Geometry: final body of the model. Coordinates: model frame, mm. A direction names the side the tool comes from. Round coordinates to 2 decimals unless told otherwise and drop trailing zeros. Loops run counter-clockwise (first coordinate to the right, second up) from the corner with the lowest first, then second, coordinate; pieces in that order, holes last. Notation, with made-up numbers: M 42,8.5 L 54,8.5 A30 ccw 54,43.5 Z; hole C 12.25,9 d9. An arc over 180 degrees is marked long. Answer as a JSON object with one key per item and string values.
from build123d import *

# Parameters (mm, degrees)
SKETCH1_W           = 100
SKETCH1_H           = 205
BOSS_EXTRUDE1_DEPTH = 3
SKETCH2_W           = 100
SKETCH2_H           = 20
BOSS_EXTRUDE2_DEPTH = 3
CUT_EXTRUDE1_REACH  = 125.257
SKETCH3_R           = 2
LPATTERN1_COUNT     = 2
LPATTERN1_PITCH     = 80
SKETCH4_W           = 100
SKETCH4_H           = 3
BOSS_EXTRUDE3_DEPTH = 15
CUT_EXTRUDE2_REACH  = 220.559
SKETCH5_R           = 1.5
LPATTERN2_COUNT     = 2
LPATTERN2_PITCH     = 80
SKETCH7_W           = 3
SKETCH7_H           = 15
CUT_EXTRUDE3_DEPTH  = 3
CUT_EXTRUDE4_REACH  = 126.021
SKETCH6_R           = 1.5


with BuildPart() as part:
    # Sketch1 → Boss-Extrude1 (new body)
    with BuildSketch(Plane(origin=(0, 0, 0), x_dir=(1, 0, 0), z_dir=(0, 1, 0))):
        Rectangle(SKETCH1_W, SKETCH1_H)
    extrude(amount=BOSS_EXTRUDE1_DEPTH)

    # Sketch2 → Boss-Extrude2 (add)
    with BuildSketch(Plane(origin=(0, 3, 0), x_dir=(1, 0, 0), z_dir=(0, 1, 0))):
        with Locations((0, 102.5)):
            Rectangle(SKETCH2_W, SKETCH2_H)
    extrude(amount=BOSS_EXTRUDE2_DEPTH)

    # Sketch3 → Cut-Extrude1 (cut, up to next)
    with BuildSketch(Plane(origin=(0, 6, 0), x_dir=(1, 0, 0), z_dir=(0, 1, 0)), mode=Mode.PRIVATE) as cut_extrude1_sk1:
        with Locations(Location((-40, 107.5, 0), (0, 0, 270))):
            Circle(SKETCH3_R)
    cut_extrude1_tool1 = extrude(cut_extrude1_sk1.sketch, amount=-CUT_EXTRUDE1_REACH, mode=Mode.PRIVATE) & part.part
    cut_extrude1 = cut_extrude1_tool1.solids().sort_by_distance((-40, 6, -107.5))[0]
    add(cut_extrude1, mode=Mode.SUBTRACT)

    # LPattern1: Cut-Extrude1 ×2
    with Locations(*[(i * LPATTERN1_PITCH, 0, 0) for i in range(1, LPATTERN1_COUNT)]):
        add(cut_extrude1, mode=Mode.SUBTRACT)

    # Sketch4 → Boss-Extrude3 (add)
    with BuildSketch(Plane(origin=(0, 3, 0), x_dir=(1, 0, 0), z_dir=(0, 1, 0))):
        with Locations((0, -98)):
            Rectangle(SKETCH4_W, SKETCH4_H)
    extrude(amount=BOSS_EXTRUDE3_DEPTH)

    # Sketch5 → Cut-Extrude2 (cut, up to next)
    with BuildSketch(Plane.XY.offset(99.5), mode=Mode.PRIVATE) as cut_extrude2_sk1:
        with Locations((-40, 10.5)):
            Circle(SKETCH5_R)
    cut_extrude2_tool1 = extrude(cut_extrude2_sk1.sketch, amount=-CUT_EXTRUDE2_REACH, mode=Mode.PRIVATE) & part.part
    cut_extrude2 = cut_extrude2_tool1.solids().sort_by_distance((-40, 10.5, 99.5))[0]
    add(cut_extrude2, mode=Mode.SUBTRACT)

    # LPattern2: Cut-Extrude2 ×2
    with Locations(*[(i * LPATTERN2_PITCH, 0, 0) for i in range(1, LPATTERN2_COUNT)]):
        add(cut_extrude2, mode=Mode.SUBTRACT)

    # Sketch7 → Cut-Extrude3 (cut)
    with BuildSketch(Plane(origin=(50, 0, 0), x_dir=(0, 0, -1), z_dir=(1, 0, 0))):
        with Locations((-98, 10.5)):
            Rectangle(SKETCH7_W, SKETCH7_H)
    extrude(amount=-CUT_EXTRUDE3_DEPTH, mode=Mode.SUBTRACT)

    # Sketch6 → Cut-Extrude4 (cut, up to next)
    with BuildSketch(Plane(origin=(0, 3, 0), x_dir=(1, 0, 0), z_dir=(0, 1, 0)), mode=Mode.PRIVATE) as cut_extrude4_sk1:
        with Locations(Location((-46, 13.97, 0), (0, 0, 270))):
            Circle(SKETCH6_R)
    cut_extrude4_tool1 = extrude(cut_extrude4_sk1.sketch, amount=-CUT_EXTRUDE4_REACH, mode=Mode.PRIVATE) & part.part
    # Sketch6 → Cut-Extrude4 (cut, up to next)
    with BuildSketch(Plane(origin=(0, 3, 0), x_dir=(1, 0, 0), z_dir=(0, 1, 0)), mode=Mode.PRIVATE) as cut_extrude4_sk2:
        with Locations(Location((46, 13.97, 0), (0, 0, 270))):
            Circle(SKETCH6_R)
    cut_extrude4_tool2 = extrude(cut_extrude4_sk2.sketch, amount=-CUT_EXTRUDE4_REACH, mode=Mode.PRIVATE) & part.part
    add(cut_extrude4_tool1.solids().sort_by_distance((-46, 3, -13.97))[0], mode=Mode.SUBTRACT)
    add(cut_extrude4_tool2.solids().sort_by_distance((46, 3, -13.97))[0], mode=Mode.SUBTRACT)


solid = part.part
1) Ray query, line 1 (X direction, y = 0.7, z = -13.97); line 2 (X direction, y = 5.1, z = -107.5); line 3 (Y direction, x = 40, z = 97). Return the intervals inside material, ascending.
Results:
{"line 1": "-50 to -47.5, -44.5 to 44.5, 47.5 to 50", "line 2": "-50 to -42, -38 to 38, 42 to 50", "line 3": "0 to 9, 12 to 18"}
2) Section query B-B (x = -27). Return the cut outline in (y, z), and give its area (3 significant figures).
Results:
{"outline": "M 0,-102.5 L 3,-102.5 L 3,-112.5 L 6,-112.5 L 6,-92.5 L 3,-92.5 L 3,96.5 L 18,96.5 L 18,99.5 L 3,99.5 L 3,102.5 L 0,102.5 Z", "area": "720 mm2"}
3) Section query C-C (y = 14.5). Return the cut outline in (x, z).
Results:
{"outline": "M -50,96.5 L 47,96.5 L 47,99.5 L -50,99.5 Z"}
4) Pin query (flat end, axial travel): P1, Ø3.5, axis at x = 2.5, y = 1, coming from the -Z side; P2, Ø10, axis at x = 4.5, y = 11, coming from the +Z side; P3, Ø3, axis at x = 32, z = 51.5, coming from the +Y side; P4, Ø2.5, axis at x = -46, z = -13.97, coming from the -Y side. Return the tip coordinate at first contact, or that it passes through.
Results:
{"P1": "z = -102.5", "P2": "z = 99.5", "P3": "y = 3", "P4": "through"}
5) Section query A-A (z = -107.5). Return the cut outline in (x, y).
Results:
{"outline": "M -50,3 L -42,3 L -42,6 L -50,6 Z; M -38,3 L 38,3 L 38,6 L -38,6 Z; M 42,3 L 50,3 L 50,6 L 42,6 Z"}
6) Section query D-D (z = -43.5). Return the cut outline in (x, y), and give its area (3 significant figures).
Results:
{"outline": "M -50,0 L 50,0 L 50,3 L -50,3 Z", "area": "300 mm2"}
7) Pull-direction query (Z, two-part tool) for faces 1 (the flat face through (50, 2, -3)), 2 (the flat face through (-1, 3, 4)), 3 (the flat face through (-2, 10, 99.5)), 4 (the cylindrical face through (-41.952, 4.521, -107.934)); classes: +Z half, -Z half, draft (parallel to the pull), parting line (faces both ways), or undercut.
Results:
{"face 1": "draft", "face 2": "undercut", "face 3": "+Z half", "face 4": "undercut"}
8) Reachability of faces 5 (the flat face through (-1, 6, -103)), 6 (the flat face through (-50, 2, 11)), 7 (the flat face through (-1, 3, -108)), 8 (the flat face through (-2, 10, 96.5)) from +Z, -Z, +X, -X, +Y, -Y: full face, straight path, thin tool, end or side. Return the list, or none.
Results:
{"face 5": "-Z, +X, -X, +Y", "face 6": "+Z, -Z, -X, +Y, -Y", "face 7": "-Z, +X, -X, -Y", "face 8": "+X, -X, +Y"}
